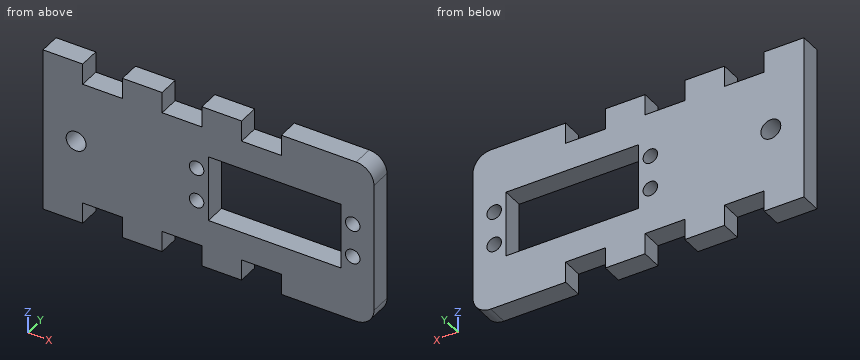
```python
from build123d import *

# Parameters (mm, degrees)
SKETCH2_R           = 2.19
SKETCH2_R_2         = 3
SKETCH2_W           = 40
SKETCH2_H           = 20
BOSS_EXTRUDE2_DEPTH = 6.35


with BuildPart() as part:
    # Sketch2 → Boss-Extrude2 (new body)
    with BuildSketch(Plane(origin=(0, 0, 0), x_dir=(1, 0, 0), z_dir=(0, 1, 0))):
        with BuildLine():
            Line((-70, 25), (-70, -25))
            Line((-70, -25), (-58, -25))
            Line((-58, -25), (-58, -18.65))
            Line((-58, -18.65), (-46, -18.65))
            Line((-46, -18.65), (-46, -25))
            Line((-46, -25), (-34, -25))
            Line((-34, -25), (-34, -18.65))
            Line((-34, -18.65), (-22, -18.65))
            Line((-22, -18.65), (-22, -25))
            Line((-22, -25), (-10, -25))
            Line((-10, -25), (-10, -18.65))
            Line((-10, -18.65), (2, -18.65))
            Line((2, -18.65), (2, -25))
            Line((2, -25), (24.62, -25))
            ThreePointArc((24.62, -25), (28.424234483, -23.424234483), (30, -19.62))
            Line((30, -19.62), (30, 19.62))
            ThreePointArc((30, 19.62), (28.424234483, 23.424234483), (24.62, 25))
            Line((24.62, 25), (2, 25))
            Line((2, 25), (2, 18.65))
            Line((2, 18.65), (-10, 18.65))
            Line((-10, 18.65), (-10, 25))
            Line((-10, 25), (-22, 25))
            Line((-22, 25), (-22, 18.65))
            Line((-22, 18.65), (-34, 18.65))
            Line((-34, 18.65), (-34, 25))
            Line((-34, 25), (-46, 25))
            Line((-46, 25), (-46, 18.65))
            Line((-46, 18.65), (-58, 18.65))
            Line((-58, 18.65), (-58, 25))
            Line((-58, 25), (-70, 25))
        make_face()
        with Locations(Location((23.59, 5.085, 0), (0, 0, 270))):
            Circle(SKETCH2_R, mode=Mode.SUBTRACT)
        with Locations(Location((23.59, -5.085, 0), (0, 0, 270))):
            Circle(SKETCH2_R, mode=Mode.SUBTRACT)
        with Locations(Location((-23.59, 5.085, 0), (0, 0, 270))):
            Circle(SKETCH2_R, mode=Mode.SUBTRACT)
        with Locations(Location((-23.59, -5.085, 0), (0, 0, 270))):
            Circle(SKETCH2_R, mode=Mode.SUBTRACT)
        with Locations(Location((-60, 0, 0), (0, 0, 270))):
            Circle(SKETCH2_R_2, mode=Mode.SUBTRACT)
        Rectangle(SKETCH2_W, SKETCH2_H, mode=Mode.SUBTRACT)
    extrude(amount=BOSS_EXTRUDE2_DEPTH)


solid = part.part
```
Verification items for the finished model (mm, model axes). Coordinates: 2 decimals unless noted, no trailing zeros. Write each loop counter-clockwise with the first axis right and the second up, starting at its lowest first coordinate (ties: lowest second). Pieces come first, ordered by that corner, then holes. Notation, with made-up numbers: M 68.5,25.5 L 114.5,25.5 A6 cw 114.5,32.5 Z; hole C -34,70.5 d7. An arc over 180 degrees is marked long. One line per item, written item: value.
Item 1: Section check D-D, the plane y = 5. State how many separate pieces and enclosed holes the cut face has, plus the area to 3 significant figures.
Check sheet entries:
separate pieces: 1
enclosed holes: 6
area: 3,640 mm^2
Item 2: Scan lines: line 1 along X through (y, z) = (5, 0); line 2 along X through (y, z) = (4.25, 5); line 3 along X through (y, z) = (2.5, -2). Record each from-to range of solid material in increasing order.
Check sheet entries:
line 1: x = -70 to -63, -57 to -20, 20 to 30
line 2: x = -70 to -25.78, -21.4 to -20, 20 to 21.4, 25.78 to 30
line 3: x = -70 to -62.24, -57.76 to -20, 20 to 30
Item 3: Section check C-C, the plane z = 9. Record the boundary of the cut face in (x, y).
Check sheet entries:
outline: M -70,0 L -20,0 L -20,6.35 L -70,6.35 Z; M 20,0 L 30,0 L 30,6.35 L 20,6.35 Z
Item 4: Section check A-A, the plane x = -60. Record the boundary of the cut face in (y, z), plus the area to 3 significant figures.
Check sheet entries:
outline: M 0,-25 L 6.35,-25 L 6.35,-3 L 0,-3 Z; M 0,3 L 6.35,3 L 6.35,25 L 0,25 Z
area: 279 mm^2
Item 5: Gauge pin test, flat ends, axial feed: pin 1 Ø1.9 at (y, z) = (3.5, -22) entering from +X; pin 2 Ø1 at (x, y) = (-28.5, 3) entering from -Z; pin 3 Ø1.9 at (x, y) = (-2, 1.5) entering from +Z; pin 4 Ø5 at (x, z) = (23.59, -5.085) entering from +Y. Record the tip position at first contact, or that the pin passes through.
Check sheet entries:
pin 1: stops at x = 29.81
pin 2: stops at z = -18.65
pin 3: stops at z = 18.65
pin 4: stops at y = 6.35
Item 6: Section check B-B, the plane x = 23.59. Record the boundary of the cut face in (y, z) (3 decimals), plus the area to 3 significant figures.
Check sheet entries:
outline: M 0,-25 L 6.35,-25 L 6.35,-7.275 L 0,-7.275 Z; M 0,-2.895 L 6.35,-2.895 L 6.35,2.895 L 0,2.895 Z; M 0,7.275 L 6.35,7.275 L 6.35,25 L 0,25 Z
area: 262 mm^2
